from build123d import *

# Parameters (mm, degrees)
BASPROSKE_W        = 13.1826
BASPROSKE_H        = 8.89
TOOTHCUT_DEPTH     = 19.216617215
TEETHCUTS_COUNT    = 12
TEETHCUTS_ANGLE    = 330
BORSKE_R           = 3.96875
BORE_DEPTH         = 13.1826508
CUT_EXTRUDE1_DEPTH = 18.974701376


with BuildPart() as part:
    # BasProSke → Base-Revolve (revolve)
    with BuildSketch(Plane(origin=(0, 0, 0), x_dir=(1, 0, 0), z_dir=(0, 1, 0)), mode=Mode.PRIVATE) as base_revolve_sk:
        with Locations((6.5913, 4.445)):
            Rectangle(BASPROSKE_W, BASPROSKE_H)
    revolve(base_revolve_sk.sketch.rotate(Axis((-10, 0, 0), (1, 0, 0)), 180), axis=Axis((-10, 0, 0), (1, 0, 0)))

    # TooCutSke → ToothCut (cut, through all)
    with BuildSketch(Plane(origin=(0, 0, 0), x_dir=(0, 0, -1), z_dir=(1, 0, 0))):
        with BuildLine():
            ThreePointArc((0.717076553, 6.002519826), (0, 6.0452), (-0.717076553, 6.002519826))
            ThreePointArc((-0.717076553, 6.002519826), (-1.069160545, 7.516029346), (-2.121611652, 8.659279483))
            ThreePointArc((-2.121611652, 8.659279483), (0, 8.9154), (2.121611652, 8.659279483))
            ThreePointArc((2.121611652, 8.659279483), (1.069160545, 7.516029346), (0.717076553, 6.002519826))
        make_face()
    toothcut = extrude(amount=TOOTHCUT_DEPTH, mode=Mode.SUBTRACT)

    # TeethCuts: ToothCut ×12 about axis
    teethcuts_axis = Axis((-10, 0, 0), (1, 0, 0))
    for i in range(1, TEETHCUTS_COUNT):
        add(toothcut.rotate(teethcuts_axis, i * TEETHCUTS_ANGLE / (TEETHCUTS_COUNT - 1)), mode=Mode.SUBTRACT)

    # BorSke → Bore (cut, symmetric)
    with BuildSketch(Plane(origin=(0, 0, 0), x_dir=(0, 0, -1), z_dir=(1, 0, 0))):
        with Locations(Location((0, 0, 0), (0, 0, 180))):
            Circle(BORSKE_R)
    extrude(amount=BORE_DEPTH, both=True, mode=Mode.SUBTRACT)

    # Sketch1 → Cut-Extrude1 (cut, through all)
    with BuildSketch(Plane(origin=(13.1826, 0, 0), x_dir=(0, 0, -1), z_dir=(1, 0, 0))):
        with BuildLine():
            Line((-1, 3.840700009), (-1, 4.71875))
            Line((-1, 4.71875), (1, 4.71875))
            Line((1, 4.71875), (1, 3.840700009))
            ThreePointArc((1, 3.840700009), (0, 3.96875), (-1, 3.840700009))
        make_face()
    extrude(amount=-CUT_EXTRUDE1_DEPTH, mode=Mode.SUBTRACT)


solid = part.part
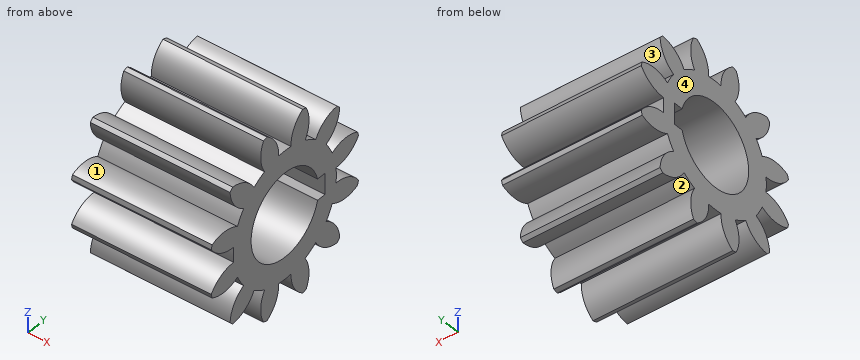
Work out the finished part from the listing and answer in its coordinate system (mm). Face numbers are marked on the shaded views. Round coordinates to 2 decimals unless told otherwise and drop trailing zeros. Loops run counter-clockwise (first coordinate to the right, second up) from the corner with the lowest first, then second, coordinate; pieces in that order, holes last. Notation, with made-up numbers: M 29.25,-9.75 L 43.25,-9.75 A16 cw 43.25,0.25 Z; hole C -31.75,82.25 d1. An arc over 180 degrees is marked long. One line per question, with ' | ' between items. Start each with the question number.
(1) A cutting plane is placed at B-B on z = 0. Write down the section's boundary in (x, y), plus the area to 3 significant figures.
(2) Flat-ended cylindrical pins translate along their axes: pin 1 Ø1 at (y, z) = (0, -6.5) entering from -X; pin 2 Ø6 at (x, z) = (11, 6.5) entering from -Y. Find the tip coordinate at first contact, or state that the pin passes through.
(3) A cutting plane is placed at C-C on z = 4.5. Write down the section's boundary in (x, y).
(4) Find the intervals of material crossed by line 1 (Z direction, x = 5.25, y = -5.75); line 2 (Y direction, x = 4, z = -5); line 3 (Z direction, x = 5.5, y = 0), in increasing order.
(5) A cutting plane is placed at A-A on y = 0. Write down the section's boundary in (x, z), plus the area to 3 significant figures.
(6) For a pull along Y with two mould halves and no side action, classify the marked faces 1, 2, 3 and 4 as released by +Y, released by -Y, zero draft, split by the parting line, or undercut.
Geometry check:
1) outline: M 0,-6.05 L 13.18,-6.05 L 13.18,-3.97 L 0,-3.97 Z; M 0,4.72 L 13.18,4.72 L 13.18,6.05 L 0,6.05 Z | area: 44.9 mm²
2) pin 1: stops at x = 0 | pin 2: stops at y = -6.44
3) outline: M 0,-5.85 L 13.18,-5.85 L 13.18,5.85 L 0,5.85 Z
4) line 1: z = -6.39 to -4.37, -2.49 to 2.49, 4.37 to 6.39 | line 2: y = -6.15 to -3.72, -3.4 to 3.4, 3.72 to 6.15 | line 3: z = -6.05 to -3.97, 3.97 to 6.05
5) outline: M 0,-6.05 L 13.18,-6.05 L 13.18,-3.97 L 0,-3.97 Z; M 0,3.97 L 13.18,3.97 L 13.18,6.05 L 0,6.05 Z | area: 54.7 mm²
6) face 1: undercut | face 2: undercut | face 3: released by +Y | face 4: zero draft
